Read the model definition and answer for the solid it produces. Units are mm, in the model's axes. Round coordinates to 2 decimals unless told otherwise and drop trailing zeros. Write each loop counter-clockwise with the first axis right and the second up, starting at its lowest first coordinate (ties: lowest second). Pieces come first, ordered by that corner, then holes.
from build123d import *

# Parameters (mm, degrees)
SKETCH1_R           = 7.5
BOSS_EXTRUDE1_DEPTH = 4


with BuildPart() as part:
    # Sketch1 → Boss-Extrude1 (new body)
    with BuildSketch(Plane(origin=(0, 0, 0), x_dir=(1, 0, 0), z_dir=(0, 1, 0))):
        with BuildLine():
            ThreePointArc((-75, -60), (-70.606601718, -70.606601718), (-60, -75))
            Line((-60, -75), (60, -75))
            ThreePointArc((60, -75), (70.606601718, -70.606601718), (75, -60))
            Line((75, -60), (75, 60))
            ThreePointArc((75, 60), (70.606601718, 70.606601718), (60, 75))
            Line((60, 75), (-60, 75))
            ThreePointArc((-60, 75), (-70.606601718, 70.606601718), (-75, 60))
            Line((-75, 60), (-75, -60))
        make_face()
        with Locations(Location((-60, -60, 0), (0, 0, 270))):
            Circle(SKETCH1_R, mode=Mode.SUBTRACT)
        with Locations(Location((-30, -60, 0), (0, 0, 270))):
            Circle(SKETCH1_R, mode=Mode.SUBTRACT)
        with Locations(Location((-60, -30, 0), (0, 0, 270))):
            Circle(SKETCH1_R, mode=Mode.SUBTRACT)
        with Locations(Location((-30, -30, 0), (0, 0, 270))):
            Circle(SKETCH1_R, mode=Mode.SUBTRACT)
        with Locations(Location((0, -30, 0), (0, 0, 270))):
            Circle(SKETCH1_R, mode=Mode.SUBTRACT)
        with Locations(Location((0, -60, 0), (0, 0, 270))):
            Circle(SKETCH1_R, mode=Mode.SUBTRACT)
        with Locations(Location((30, -60, 0), (0, 0, 270))):
            Circle(SKETCH1_R, mode=Mode.SUBTRACT)
        with Locations(Location((60, -60, 0), (0, 0, 270))):
            Circle(SKETCH1_R, mode=Mode.SUBTRACT)
        with Locations(Location((30, -30, 0), (0, 0, 270))):
            Circle(SKETCH1_R, mode=Mode.SUBTRACT)
        with Locations(Location((60, -30, 0), (0, 0, 270))):
            Circle(SKETCH1_R, mode=Mode.SUBTRACT)
        with Locations(Location((-60, 0, 0), (0, 0, 270))):
            Circle(SKETCH1_R, mode=Mode.SUBTRACT)
        with Locations(Location((-60, 30, 0), (0, 0, 270))):
            Circle(SKETCH1_R, mode=Mode.SUBTRACT)
        with Locations(Location((-30, 0, 0), (0, 0, 270))):
            Circle(SKETCH1_R, mode=Mode.SUBTRACT)
        with Locations(Location((0, 0, 0), (0, 0, 270))):
            Circle(SKETCH1_R, mode=Mode.SUBTRACT)
        with Locations(Location((-30, 30, 0), (0, 0, 270))):
            Circle(SKETCH1_R, mode=Mode.SUBTRACT)
        with Locations(Location((0, 30, 0), (0, 0, 270))):
            Circle(SKETCH1_R, mode=Mode.SUBTRACT)
        with Locations(Location((-60, 60, 0), (0, 0, 270))):
            Circle(SKETCH1_R, mode=Mode.SUBTRACT)
        with Locations(Location((-30, 60, 0), (0, 0, 270))):
            Circle(SKETCH1_R, mode=Mode.SUBTRACT)
        with Locations(Location((0, 60, 0), (0, 0, 270))):
            Circle(SKETCH1_R, mode=Mode.SUBTRACT)
        with Locations(Location((30, 0, 0), (0, 0, 270))):
            Circle(SKETCH1_R, mode=Mode.SUBTRACT)
        with Locations(Location((30, 30, 0), (0, 0, 270))):
            Circle(SKETCH1_R, mode=Mode.SUBTRACT)
        with Locations(Location((60, 0, 0), (0, 0, 270))):
            Circle(SKETCH1_R, mode=Mode.SUBTRACT)
        with Locations(Location((60, 30, 0), (0, 0, 270))):
            Circle(SKETCH1_R, mode=Mode.SUBTRACT)
        with Locations(Location((30, 60, 0), (0, 0, 270))):
            Circle(SKETCH1_R, mode=Mode.SUBTRACT)
        with Locations(Location((60, 60, 0), (0, 0, 270))):
            Circle(SKETCH1_R, mode=Mode.SUBTRACT)
    extrude(amount=BOSS_EXTRUDE1_DEPTH)


solid = part.part
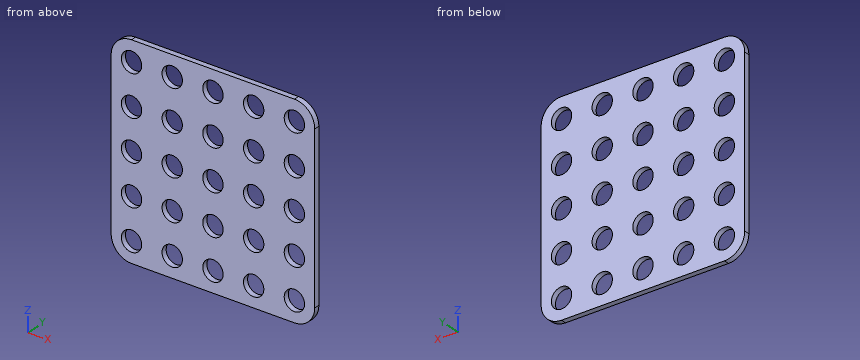
Q1. Section C-C (y = 3.25) is taken. State how many separate pieces and enclosed holes the cut face has, then the cut area to 3 significant figures.
Verdict:
separate pieces: 1
enclosed holes: 25
area: 17,900 mm2
Q2. A flat-ended cylindrical pin translates along its axis: pin 1 Ø13.5 at (x, z) = (30, 0) entering from +Y. Find the tip coordinate at first contact, or state that the pin passes through.
Verdict:
pin 1: passes through
Q3. Straight lines are drawn through the part: probe 1 along X at (y, z) = (1.1, 30); probe 2 along X at (y, z) = (0.35, 29); probe 3 along Z at (x, y) = (61, 2). For each, find the intervals that lie inside material, in ascending order.
Verdict:
probe 1: x = -75 to -67.5, -52.5 to -37.5, -22.5 to -7.5, 7.5 to 22.5, 37.5 to 52.5, 67.5 to 75
probe 2: x = -75 to -67.43, -52.57 to -37.43, -22.57 to -7.43, 7.43 to 22.57, 37.43 to 52.57, 67.43 to 75
probe 3: z = -74.97 to -67.43, -52.57 to -37.43, -22.57 to -7.43, 7.43 to 22.57, 37.43 to 52.57, 67.43 to 74.97
Q4. Section A-A (x = 0) is taken. Determine the outline of the cut face in (y, z), then the cut area to 3 significant figures.
Verdict:
outline: (0, -75) - (4, -75) - (4, -67.5) - (0, -67.5) - close; (0, -52.5) - (4, -52.5) - (4, -37.5) - (0, -37.5) - close; (0, -22.5) - (4, -22.5) - (4, -7.5) - (0, -7.5) - close; (0, 7.5) - (4, 7.5) - (4, 22.5) - (0, 22.5) - close; (0, 37.5) - (4, 37.5) - (4, 52.5) - (0, 52.5) - close; (0, 67.5) - (4, 67.5) - (4, 75) - (0, 75) - close
area: 300 mm2
Q5. Section B-B (z = 0) is taken. Determine the outline of the cut face in (x, y), then the cut area to 3 significant figures.
Verdict:
outline: (-75, 0) - (-67.5, 0) - (-67.5, 4) - (-75, 4) - close; (-52.5, 0) - (-37.5, 0) - (-37.5, 4) - (-52.5, 4) - close; (-22.5, 0) - (-7.5, 0) - (-7.5, 4) - (-22.5, 4) - close; (7.5, 0) - (22.5, 0) - (22.5, 4) - (7.5, 4) - close; (37.5, 0) - (52.5, 0) - (52.5, 4) - (37.5, 4) - close; (67.5, 0) - (75, 0) - (75, 4) - (67.5, 4) - close
area: 300 mm2
